```python
from build123d import *

# Parameters (mm, degrees)
CYLINDER062_R          = 1.25
CYLINDER062_DEPTH      = 10
CYLINDER060_R          = 1.25
CYLINDER060_DEPTH      = 10
CYLINDER061_R          = 1.25
CYLINDER061_DEPTH      = 10
CYLINDER059_R          = 1.25
CYLINDER059_DEPTH      = 10
BOX025_W               = 10
BOX025_H               = 8
BOX025_DEPTH           = 20
BOX026_W               = 10
BOX026_H               = 15
BOX026_DEPTH           = 5
BOX024_W               = 10
BOX024_H               = 15
BOX024_DEPTH           = 5
CUT030_PLACEMENT_ANGLE = 90


with BuildPart() as cylinder062:
    # Cylinder062 → Cylinder062 (new body)
    with BuildSketch(Plane(origin=(87.5, 61, 14), x_dir=(1, 0, 0), z_dir=(0, -1, 0))):
        Circle(CYLINDER062_R)
    extrude(amount=CYLINDER062_DEPTH)


with BuildPart() as fusion060:
    # Cylinder060 → Cylinder060 (new body)
    with BuildSketch(Plane(origin=(87.5, 11, 14), x_dir=(1, 0, 0), z_dir=(0, -1, 0))):
        Circle(CYLINDER060_R)
    extrude(amount=CYLINDER060_DEPTH)

    # Fusion060: union Cylinder062
    add(cylinder062.part)


with BuildPart() as cylinder061:
    # Cylinder061 → Cylinder061 (new body)
    with BuildSketch(Plane(origin=(82.5, 61, 14), x_dir=(1, 0, 0), z_dir=(0, -1, 0))):
        Circle(CYLINDER061_R)
    extrude(amount=CYLINDER061_DEPTH)


with BuildPart() as fusion061:
    # Cylinder059 → Cylinder059 (new body)
    with BuildSketch(Plane(origin=(82.5, 11, 14), x_dir=(1, 0, 0), z_dir=(0, -1, 0))):
        Circle(CYLINDER059_R)
    extrude(amount=CYLINDER059_DEPTH)

    # Fusion062: union Cylinder061
    add(cylinder061.part)

    # Fusion061: union Fusion060
    add(fusion060.part)


with BuildPart() as fusion061_1:
    # Fusion061 placement: moved
    add(fusion061.part.moved(Location((0, -10, 0))))


with BuildPart() as cube004:
    # Box025 → Box025 (new body)
    with BuildSketch(Plane(origin=(0, -10, 0), x_dir=(1, 0, 0), z_dir=(0, 0, 1))):
        with Locations((5, 4)):
            Rectangle(BOX025_W, BOX025_H)
    extrude(amount=BOX025_DEPTH)


with BuildPart() as cube005:
    # Box026 → Box026 (new body)
    with BuildSketch(Plane(origin=(0, -10, 20), x_dir=(1, 0, 0), z_dir=(0, 0, 1))):
        with Locations((5, 7.5)):
            Rectangle(BOX026_W, BOX026_H)
    extrude(amount=BOX026_DEPTH)


with BuildPart() as cut030:
    # Box024 → Box024 (new body)
    with BuildSketch(Plane(origin=(0, -10, -5), x_dir=(1, 0, 0), z_dir=(0, 0, 1))):
        with Locations((5, 7.5)):
            Rectangle(BOX024_W, BOX024_H)
    extrude(amount=BOX024_DEPTH)

    # Fusion066: union Cube004, Cube005
    add(cube004.part)
    add(cube005.part)


with BuildPart() as cut030_1:
    # Fusion066 placement: moved
    add(cut030.part.moved(Location((80, 2, 0))))

    # Cut030: cut Fusion061
    add(fusion061_1.part, mode=Mode.SUBTRACT)


with BuildPart() as cut030_2:
    # Cut030 placement: moved
    add(cut030_1.part.moved(Location((0, -10, 0))).rotate(Axis((0, -10, 0), (1, 0, 0)), CUT030_PLACEMENT_ANGLE))


solid = cut030_2.part
```
Verification items for the finished model (mm, model axes). A direction names the side the tool comes from. Round coordinates to 2 decimals unless told otherwise and drop trailing zeros. Write each loop counter-clockwise with the first axis right and the second up, starting at its lowest first coordinate (ties: lowest second). Pieces come first, ordered by that corner, then holes. Notation, with made-up numbers: (32.5, 4.5) - (78.5, 4.5) arc R23 cw to (78.5, 38.5) - close; hole circle Ø2 at (35.25, 25). An arc over 180 degrees is marked (long way). Answer as a JSON object with one key per item and string values. Group by question number.
Q1. Go/stop test with a flat-tipped pin: pin 1 Ø3 at (x, y) = (87, -21) entering from +Z. Record where the tip stops, or that it passes through.
Q2. Section check A-A, the plane y = -24. Enter the section's corners in (x, z), plus the area to 3 significant figures.
Q3. Mould release check, pull along Y, two halves, no side actions. Record for faces 3 (the flat face through (85, -35, 0)), 4 (the flat face through (85, -20, 0)), 5 (the flat face through (90, -20, -2)): released by +Y, released by -Y, zero draft, split by the parting line, or undercut.
Q4. Section check D-D, the plane z = -6.25. Enter the section's corners in (x, y).
Q5. Thickness scan on line 1 (Y direction, x = 82.5, z = -5.25); line 2 (Y direction, x = 87.5, z = 5.25); line 3 (Z direction, x = 89, y = -15.5). Record the ranges inside material, lowest first.
Q6. Section check B-B, the plane x = 82.5. Enter the section's corners in (y, z).
Q7. Tool access check on faces 1 (the flat face through (85, -10, 4)), 2 (the cylindrical face through (83.655, -23.521, -3.944)). Record the directions out of +Z, -Z, +X, -X, +Y, -Y that give a thin tool (end or side, any length) a straight path to the whole face; none if there is none.
Q8. Section check C-C, the plane z = 3. Enter the section's corners in (x, y), plus the area to 3 significant figures.
Found:
{
 "1": {"pin 1": "stops at z = 0"},
 "2": {"outline": "(80, -8) - (81.25, -8) - (81.25, 0) - (80, 0) - close; (83.75, -8) - (86.25, -8) - (86.25, 0) - (83.75, 0) - close; (88.75, -8) - (90, -8) - (90, 0) - (88.75, 0) - close", "area": "40.0 mm^2"},
 "3": {"face 3": "released by -Y", "face 4": "undercut", "face 5": "zero draft"},
 "4": {"outline": "(80, -35) - (90, -35) - (90, -5) - (80, -5) - close; hole circle Ø2.5 at (82.5, -24); hole circle Ø2.5 at (87.5, -24)"},
 "5": {"line 1": "y = -35 to -25.25, -22.75 to -5", "line 2": "y = -35 to -30, -10 to -5", "line 3": "z = -8 to 0"},
 "6": {"outline": "(-35, -8) - (-25.25, -8) - (-25.25, 0) - (-30, 0) - (-30, 7) - (-35, 7) - close; (-22.75, -8) - (-5, -8) - (-5, 7) - (-10, 7) - (-10, 0) - (-22.75, 0) - close"},
 "7": {"face 1": "+Z, +X, -X", "face 2": "+Z, -Z"},
 "8": {"outline": "(80, -35) - (90, -35) - (90, -30) - (80, -30) - close; (80, -10) - (90, -10) - (90, -5) - (80, -5) - close", "area": "100 mm^2"}
}
